Read the model definition and answer for the solid it produces. Units are mm, in the model's axes. Face numbers are marked on the shaded views. A direction names the side the tool comes from. Give positions to 0.01 mm unless a question says otherwise; leave off trailing zeros. Loops run counter-clockwise (first coordinate to the right, second up) from the corner with the lowest first, then second, coordinate; pieces in that order, holes last. Notation, with made-up numbers: (24, 49.25) - (39, 49.25) arc R11 cw to (39, 67.25) - close; hole circle Ø4 at (12, 33). An arc over 180 degrees is marked (long way). Use a Markdown table: item, result. Add a question column.
Item 1: Which of the six approach directions +Z, -Z, +X, -X, +Y, -Y give full straight-line access (tool end or side, diameter ignored) to the marked faces 1, 2 and 3?
Item 2: Consider probe 1 along Z at (x, y) = (-12, 15.5); probe 2 along Z at (x, y) = (-6, 18); probe 3 along Z at (x, y) = (17.5, 14). Determine where each line is inside the solid, lowest interval first. Write a range as [from, to].
Item 3: A cutting plane is placed at C-C (z = -57). Determine the outline of the cut face in (x, y), plus the area to 3 significant figures.
Item 4: Each of these flat-tipped pins is pushed along its axis until it touches: P1, Ø2, axis at x = -8, z = -179, coming from the +Y side (3 decimals); P2, Ø3, axis at x = -1, y = -17.5, coming from the -Z side; P3, Ø1, axis at y = -19, z = -48, coming from the +X side; P4, Ø2, axis at x = -3.5, y = 20, coming from the -Z side. Where does it stop, or does it pass through?
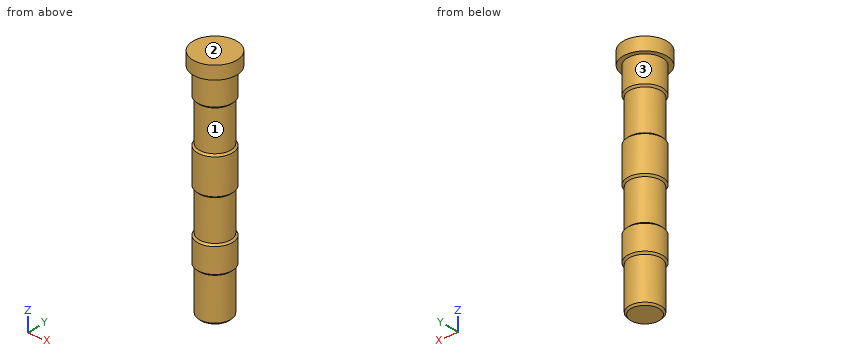
Autodesk Inventor part; units mm, degrees
ref_plane "YZ Plane" through (0, 0, 0) normal (1, 0, 0) x (0, 1, 0)
ref_plane "XZ Plane" through (0, 0, 0) normal (0, 1, 0) x (-1, 0, 0)
ref_plane "XY Plane" through (0, 0, 0) normal (0, 0, 1) x (1, 0, 0)
sketch "Эскиз1" plane through (0, 0, 0) normal (0, 0, 1) x (1, 0, 0)
  circle A0 centre (0, 0) radius 25
  dimension "d0" = 50
extrude "Выдавливание1" add sketch "Эскиз1" along normal blind 15
sketch "Эскиз2" plane through (0, 0, 0) normal (0, 0, -1) x (-1, 0, 0)
  circle A0 centre (0, 0) radius 25
  circle A1 centre (0, 0) radius 20
  dimension "d3" = 40
extrude "Выдавливание2" add sketch "Эскиз2" along normal blind 200 contours A1
sketch "Эскиз3" plane through (0, 0, 0) normal (1, 0, 0) x (0, 1, 0)
  line L0 (-20, -200) -> (20, -200)
  line L1 (20, 0) -> (-20, 0)
  line L2 (20, 0) -> (20, -200)
  line L3 (-20, 0) -> (-20, -200)
  line L4 (20, 0) -> (20, -30)
  line L5 (20, -30) -> (20, -30)
  line L6 (18, -32) -> (18, -78)
  line L7 (20, -80) -> (20, -80)
  line L8 (20, -80) -> (20, -120)
  line L9 (20, -120) -> (20, -120)
  line L10 (18, -122) -> (18, -168)
  line L11 (20, -170) -> (20, -170)
  line L12 (20, -30) -> (18, -32)
  line L13 (18, -78) -> (20, -80)
  line L14 (20, -120) -> (18, -122)
  line L15 (18, -168) -> (20, -170)
  line L16 (0, 0) -> (0, -14)
  line L17 (20, -200) -> (18, -200)
  line L18 (-20, -200) -> (20, -200)
  line L19 (18, -200) -> (20, -198)
  line L20 (20, 0) -> (20, -200)
  point P0 (18, -30)
  point P1 (18, -80)
  point P2 (18, -120)
  point P3 (18, -170)
  dimension "d6" = 30
  dimension "d7" = 2
  dimension "d8" = 50
  dimension "d9" = 40
  dimension "d10" = 50
  dimension "d11" = 2
  dimension "d12" = 2
  dimension "d13" = 2
  dimension "d14" = 2
  dimension "d15" = 2
  dimension "d16" = 2
  dimension "d17" = 2
  dimension "d18" = 2
  dimension "d27" = 2
revolve "Вращение1" cut sketch "Эскиз3" angle 360 about axis through (0, 0, 0) along (0, 0, -1) contours L19 L2 L0 | L15 L10 L14 L2 | L2 L13 L6 L12
sketch "Эскиз5" plane through (0, 0, -200) normal (0, 0, -1) x (-1, 0, 0)
  circle A0 centre (0, 0) radius 18
extrude "Выдавливание4" add sketch "Эскиз5" along normal blind 50
thread "Резьба2"
chamfer "Фаска2" distance 2 angle 45 1 edges at (18, 0, -250)
properties part number "Болт шатуна" material "Сталь, высокопрочная, низколегированная"
Geometry says:
| question | item | result |
|---|---|---|
| 1 | face 1 | none |
| 1 | face 2 | +Z, +X, -X, +Y, -Y |
| 1 | face 3 | -Z |
| 2 | probe 1 | [-198.4, -169.6], [-120.4, -79.6], [-30.4, 15] |
| 2 | probe 2 | [-199.03, -168.97], [-121.03, -78.97], [-31.03, 15] |
| 2 | probe 3 | [0, 15] |
| 3 | outline | circle Ø36 at (0, 0) |
| 3 | area | 1,020 mm² |
| 4 | P1 | y = 18.735 |
| 4 | P2 | z = -249.97 |
| 4 | P3 | through |
| 4 | P4 | z = -198.7 |
